The listing builds one solid part. Answer for the finished solid, in the listing's coordinates (mm). A direction names the side the tool comes from. Give positions to 0.01 mm unless a question says otherwise; leave off trailing zeros. Write each loop counter-clockwise with the first axis right and the second up, starting at its lowest first coordinate (ties: lowest second). Pieces come first, ordered by that corner, then holes. Notation, with made-up numbers: (89.5, 86.5) -> (133.5, 86.5) arc R14 cw to (133.5, 104.5) -> close; hole circle Ø1 at (-34.5, 65.5). An arc over 180 degrees is marked (long way). Use CSV: the item, a comma, the result in double quotes. Start each with the question number.
from build123d import *

# Parameters (mm, degrees)
EXTRUDE_1_DEPTH = 3


with BuildPart() as part:
    # 草图1 → 凸台-拉伸1 (new body)
    with BuildSketch(Plane.XY):
        Polygon((-25, -10), (-20, -10), (-20, -13), (-10, -13), (-10, -10), (-5, -10), (-5, -13), (5, -13), (5, -10), (10, -10), (10, -13), (20, -13), (20, -10), (25, -10), (25, -8), (25, -2), (25, 2), (25, 8), (25, 10), (20, 10), (20, 13), (10, 13), (10, 10), (5, 10), (5, 13), (-5, 13), (-5, 10), (-10, 10), (-10, 13), (-20, 13), (-20, 10), (-25, 10), (-25, 8), (-25, 2), (-25, -2), (-25, -8), align=None)
        Polygon((-12.5, 7), (12.5, 7), (0, 2), align=None, mode=Mode.SUBTRACT)
        Polygon((20, -5), (20, 5), (7.5, 0), align=None, mode=Mode.SUBTRACT)
        Polygon((-12.5, -7), (12.5, -7), (0, -2), align=None, mode=Mode.SUBTRACT)
        Polygon((-20, -5), (-7.5, 0), (-20, 5), align=None, mode=Mode.SUBTRACT)
    extrude(amount=EXTRUDE_1_DEPTH)


solid = part.part
Q1. The mould has two halves that part along X. Classify faces 6 (the face through (15, -13, 1)), 7 (the face through (8, 10, 1)), 8 (the face through (-25, 0, 1)), 9 (the face through (0, 7, 1)): +X half, -X half, draft (parallel to the pull), parting line (faces both ways), or undercut.
Q2. Section D-D on x = 12 is taken. Give the vertices of the cut face in (y, z), then the cut area to 3 significant figures.
Q3. Straight lines are drawn through the part: L1, parallel to X at y = -11, z = 0.5; L2, parallel to Y at x = -0.5, z = 0.95; L3, parallel to Y at x = 2, z = 1.3. For each, find the intervals that lie inside material, in ascending order.
Q4. Section B-B on y = -0.5 is taken. Give the vertices of the cut face in (x, z).
Q5. For faces 1 (the face through (0, 0, 3)), 2 (the face through (-10, 11, 1)), 3 (the face through (-5, -11, 1)), 4 (the face through (0, 0, 0)), 5 (the face through (-6.163, 4.465, 1.479)), determine the directions among +Z, -Z, +X, -X, +Y, -Y from which every point of the face is accessible in a straight line to the end or side of a thin tool.
Q6. Section A-A on x = -18 is taken. Give the vertices of the cut face in (y, z).
Q7. Flat-ended cylindrical pins translate along their axes: pin 1 Ø1.5 at (y, z) = (11.5, 1) entering from +X; pin 2 Ø1.5 at (y, z) = (11.5, 1.5) entering from -X; pin 3 Ø10 at (x, y) = (13.5, -4) entering from -Z. Find the tip coordinate at first contact, or state that the pin passes through.
Q8. Section C-C on x = -1 is taken. Give the vertices of the cut face in (y, z), then the cut area to 3 significant figures.
Output:
1,face 6,"draft"
1,face 7,"undercut"
1,face 8,"-X half"
1,face 9,"undercut"
2,outline,"(-13, 0) -> (-7, 0) -> (-7, 3) -> (-13, 3) -> close; (-6.8, 0) -> (-1.8, 0) -> (-1.8, 3) -> (-6.8, 3) -> close; (1.8, 0) -> (6.8, 0) -> (6.8, 3) -> (1.8, 3) -> close; (7, 0) -> (13, 0) -> (13, 3) -> (7, 3) -> close"
2,area,"66.0 mm²"
3,L1,"-20 to -10, -5 to 5, 10 to 20"
3,L2,"-13 to -7, -2.2 to 2.2, 7 to 13"
3,L3,"-13 to -7, -2.8 to 2.8, 7 to 13"
4,outline,"(-25, 0) -> (-20, 0) -> (-20, 3) -> (-25, 3) -> close; (-8.75, 0) -> (8.75, 0) -> (8.75, 3) -> (-8.75, 3) -> close; (20, 0) -> (25, 0) -> (25, 3) -> (20, 3) -> close"
5,face 1,"+Z, +X, -X, +Y, -Y"
5,face 2,"+Z, -Z, +Y"
5,face 3,"+Z, -Z, -Y"
5,face 4,"-Z, +X, -X, +Y, -Y"
5,face 5,"+Z, -Z"
6,outline,"(-13, 0) -> (-4.2, 0) -> (-4.2, 3) -> (-13, 3) -> close; (4.2, 0) -> (13, 0) -> (13, 3) -> (4.2, 3) -> close"
7,pin 1,"x = 20"
7,pin 2,"x = -20"
7,pin 3,"z = 0"
8,outline,"(-13, 0) -> (-7, 0) -> (-7, 3) -> (-13, 3) -> close; (-2.4, 0) -> (2.4, 0) -> (2.4, 3) -> (-2.4, 3) -> close; (7, 0) -> (13, 0) -> (13, 3) -> (7, 3) -> close"
8,area,"50.4 mm²"
